from build123d import *

# Parameters (mm, degrees)
SKETCH1_R           = 40
SKETCH1_R_2         = 37
EXTRUDE_THIN1_DEPTH = 150
SKETCH2_R           = 38
SKETCH2_R_2         = 36
EXTRUDE_THIN2_DEPTH = 74
SKETCH7_R           = 38
SKETCH7_R_2         = 37
EXTRUDE_THIN7_DEPTH = 74
SKETCH4_R           = 38
SKETCH4_R_2         = 36
BOSS_EXTRUDE2_DEPTH = 224


with BuildPart() as part:
    # Sketch1 → Extrude-Thin1 (new body)
    with BuildSketch(Plane(origin=(0, 0, 0), x_dir=(1, 0, 0), z_dir=(0, 1, 0))):
        Circle(SKETCH1_R)
        Circle(SKETCH1_R_2, mode=Mode.SUBTRACT)
    extrude(amount=EXTRUDE_THIN1_DEPTH)



with BuildPart() as body_2:
    # Sketch2 → Extrude-Thin2 (new body)
    with BuildSketch(Plane.XZ):
        Circle(SKETCH2_R)
        Circle(SKETCH2_R_2, mode=Mode.SUBTRACT)
    extrude(amount=EXTRUDE_THIN2_DEPTH)


with BuildPart() as body_3:
    # Sketch7 → Extrude-Thin7 (new body)
    with BuildSketch(Plane(origin=(0, 150, 0), x_dir=(1, 0, 0), z_dir=(0, 1, 0))):
        Circle(SKETCH7_R)
        Circle(SKETCH7_R_2, mode=Mode.SUBTRACT)
    extrude(amount=EXTRUDE_THIN7_DEPTH)


with BuildPart() as part_1:
    add(part.part)

    add(body_2.part)  # Boss-Extrude2 merges body 2

    add(body_3.part)  # Boss-Extrude2 merges body 3
    # Sketch4 → Boss-Extrude2 (add, through all)
    with BuildSketch(Plane(origin=(0, 0, 0), x_dir=(1, 0, 0), z_dir=(0, 1, 0))):
        with Locations(Location((0, 0, 0), (0, 0, 90))):
            Circle(SKETCH4_R)
        with Locations(Location((0, 0, 0), (0, 0, 90))):
            Circle(SKETCH4_R_2, mode=Mode.SUBTRACT)
    extrude(amount=BOSS_EXTRUDE2_DEPTH)


solid = part_1.part
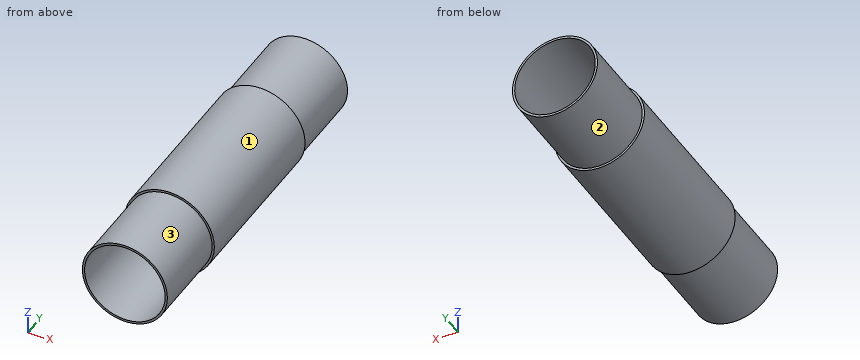
The model under review builds one solid part; all positions refer to its coordinate system, in mm. Face numbers are marked on the shaded views. A direction names the side the tool comes from. Give positions to 0.01 mm unless a question says otherwise; leave off trailing zeros. Loops run counter-clockwise (first coordinate to the right, second up) from the corner with the lowest first, then second, coordinate; pieces in that order, holes last. Notation, with made-up numbers: (47.5, 56) -> (76.5, 56) arc R24 ccw to (76.5, 68) -> close; hole circle Ø10 at (70.25, 88). An arc over 180 degrees is marked (long way). Put each result on its own line as item: value. Start each with the question number.
1. Clearance check with flat-ended pins moving along their axes: P1, Ø4, axis at y = 104.5, z = -10, coming from the +X side; P2, Ø10, axis at x = -18.5, y = 99.5, coming from the -Z side; P3, Ø4, axis at y = 5.5, z = 16, coming from the -X side. State where each tip first meets the part, or that it passes through.
2. We need section A-A on z = 0. State the section outline as (x, y) points, then the cut area to 3 significant figures.
3. We need section C-C on y = 135. State the section outline as (x, z) points, then the cut area to 3 significant figures.
4. For the marked faces 1, 2 and 3, list the 3-axis set-ups (+Z, -Z, +X, -X, +Y, -Y) from which the entire face can be reached by the end or side of a thin tool; tool diameter is ignored.
5. We need section B-B on x = 0. State the section outline as (y, z) points.
6. Wall thickness on probe 1 along X at (y, z) = (-17, 0); probe 2 along X at (y, z) = (115, 0): over which ranges is each line inside the solid? List them lowest first.
Determined:
1. P1: x = 39.19
1. P2: z = -37.65
1. P3: x = -37.47
2. outline: (-40, 0) -> (-38, 0) -> (-38, -74) -> (-36, -74) -> (-36, 224) -> (-38, 224) -> (-38, 150) -> (-40, 150) -> close; (36, -74) -> (38, -74) -> (38, 0) -> (40, 0) -> (40, 150) -> (38, 150) -> (38, 224) -> (36, 224) -> close
2. area: 1,790 mm^2
3. outline: circle Ø80 at (0, 0); hole circle Ø72 at (0, 0)
3. area: 955 mm^2
4. face 1: +Y, -Y
4. face 2: +Y
4. face 3: -Y
5. outline: (-74, -38) -> (0, -38) -> (0, -40) -> (150, -40) -> (150, -38) -> (224, -38) -> (224, -36) -> (-74, -36) -> close; (-74, 36) -> (224, 36) -> (224, 38) -> (150, 38) -> (150, 40) -> (0, 40) -> (0, 38) -> (-74, 38) -> close
6. probe 1: -38 to -36, 36 to 38
6. probe 2: -40 to -36, 36 to 40
